```python
from build123d import *

# Parameters (mm, degrees)
ESQUISSE2_R                  = 76
ESQUISSE2_R_2                = 74.5
BOSS_EXTRU_1_DEPTH           = 138
ENL_V_MAT_EXTRU_1_DEPTH      = 639.853172531
ENL_V_MAT_EXTRU_1_DEPTH_BACK = 639.853172531
ESQUISSE3_R                  = 2.5
ESQUISSE4_R                  = 4
ENL_V_MAT_EXTRU_2_DEPTH      = 639.853172531


with BuildPart() as part:
    # Esquisse1 → Révolution3 (revolve)
    with BuildSketch(Plane.XY, mode=Mode.PRIVATE) as r_volution3_sk:
        with BuildLine():
            Line((-491.50407149, 74.5), (-490.50407149, 74.5))
            add(Edge.make_bspline(
                [(-490.50407149, 74.5), (-210.641164775, 74.5), (88.162014774, 0)],
                knots=[0, 0, 0, 1, 1, 1], degree=2))
            Line((88.162014774, 0), (98.49592851, 0))
            Line((98.49592851, 0), (88.766819513, 2.425739316))
            add(Edge.make_bspline(
                [(-490.50407149, 77), (-484.660460903, 77), (-472.982345417, 76.951439725), (-449.554479537, 76.660081056), (-420.185100497, 75.931692001), (-384.790988872, 74.474939228), (-337.4032762, 71.755715065), (-277.799454783, 66.900072587), (-205.68518197, 58.742907607), (-132.981039596, 48.255507982), (-71.903167077, 37.574386444), (-22.745510555, 27.864426733), (14.268518345, 19.999918851), (45.241417883, 12.959556247), (70.082061744, 7.038903949), (82.547637876, 3.976355453), (88.766819513, 2.425739316)],
                knots=[0, 0, 0, 0, 0.03125, 0.0625, 0.125, 0.1875, 0.25, 0.375, 0.5, 0.625, 0.75, 0.8125, 0.875, 0.9375, 0.96875, 1, 1, 1, 1], degree=3))
            Line((-490.50407149, 77), (-491.50407149, 77))
            Line((-491.50407149, 77), (-491.50407149, 74.5))
        make_face()
    revolve(r_volution3_sk.sketch.rotate(Axis((-218.288054544, 0, 0), (1, 0, 0)), 90), axis=Axis((-218.288054544, 0, 0), (1, 0, 0)))

    # Esquisse2 → Boss.-Extru.1 (add)
    with BuildSketch(Plane.ZY.offset(491.50407149)):
        with Locations(Location((0, 0, 0), (0, 0, 180))):
            Circle(ESQUISSE2_R)
        Circle(ESQUISSE2_R_2, mode=Mode.SUBTRACT)
    extrude(amount=BOSS_EXTRU_1_DEPTH)

    # Esquisse3 → Enlèv. mat.-Extru.1 (cut, two sides: drawn at the far end of the back side and taken through both)
    with BuildSketch(Plane(origin=(0, 0, 0), x_dir=(1, 0, 0), z_dir=(0, 1, 0)).offset(-ENL_V_MAT_EXTRU_1_DEPTH_BACK)):
        with Locations(Location((-486.50407149, 0, 0), (0, 0, 270))):
            Circle(ESQUISSE3_R)
    extrude(amount=ENL_V_MAT_EXTRU_1_DEPTH + ENL_V_MAT_EXTRU_1_DEPTH_BACK, mode=Mode.SUBTRACT)

    # Esquisse4 → Enlèv. mat.-Extru.2 (cut, through all)
    with BuildSketch(Plane(origin=(0, 0, 0), x_dir=(0, 0, -1), z_dir=(1, 0, 0))):
        with Locations(Location((0, 0, 0), (0, 0, 180))):
            Circle(ESQUISSE4_R)
    extrude(amount=ENL_V_MAT_EXTRU_2_DEPTH, mode=Mode.SUBTRACT)


solid = part.part
```
Can you work these out from the model? Positions are in its coordinate system, mm. A direction names the side the tool comes from. Coordinates: 2 decimals unless noted, no trailing zeros.
Item 1: Please list where these lines run through material, in increasing order: L1, parallel to Y at x = -491, z = 0; L2, parallel to Z at x = -133.5, y = -41; L3, parallel to Y at x = -322, z = 59.
Answers below:
L1: y = -77 to -74.5, 74.5 to 77
L2: z = -24.89 to -19.58, 19.58 to 24.89
L3: y = -38.39 to -33.57, 33.57 to 38.39
Item 2: Which directions (+Z, -Z, +X, -X, +Y, -Y) give clear straight access to the entire face, cutting with the end or side of a thin tool? Please do faces 1 (the face through (-629.504, 50, -56)), 2 (the face through (-559.54, 74.19, 16.48)).
Answers below:
face 1: +Z, -Z, -X, +Y, -Y
face 2: -X
Item 3: I'm going to push flat-ended pins straight in: pin 1 (2 mm diameter, centred on x = -364.5, z = 27, fed in from -Y); pin 2 (5 mm diameter, centred on x = -242, y = -48, fed in from -Z); pin 3 (6 mm diameter, centred on x = -276, y = -16.5, fed in from +Z). Where does each tip first touch, or does it pass through?
Answers below:
pin 1: stops at y = -68.52
pin 2: stops at z = -43.25
pin 3: stops at z = 65.03
